Can you work these out from the model? Positions are in its coordinate system, mm. Face numbers are marked on the shaded views. A direction names the side the tool comes from. Give positions to 0.01 mm unless a question says otherwise; leave off trailing zeros. Write each loop counter-clockwise with the first axis right and the second up, starting at its lowest first coordinate (ties: lowest second). Pieces come first, ordered by that corner, then holes.
from build123d import *

# Parameters (mm, degrees)
SKETCH1_R             = 12.7
BOSS_EXTRUDE1_DEPTH   = 6.35
SKETCH2_R             = 6.35
CUT_EXTRUDE1_DEPTH    = 2.38125
SKETCH3_R             = 3.1115
CUT_EXTRUDE2_DEPTH    = 3.175
SKETCH4_R             = 1.190625
CUT_EXTRUDE3_DEPTH    = 4.96875
F_6_32_TAPPED_HOLE1_D = 2.7051
SKETCH7_R             = 1.778
CUT_EXTRUDE4_DEPTH    = 7.35
SKETCH8_R             = 3.175
CUT_EXTRUDE5_DEPTH    = 3.175
CIRPATTERN2_COUNT     = 4
FILLET1_R             = 1.5875


with BuildPart() as part:
    # Sketch1 → Boss-Extrude1 (new body)
    with BuildSketch(Plane(origin=(0, 0, 0), x_dir=(1, 0, 0), z_dir=(0, 1, 0))):
        Circle(SKETCH1_R)
    extrude(amount=BOSS_EXTRUDE1_DEPTH)

    # Sketch2 → Cut-Extrude1 (cut)
    with BuildSketch(Plane(origin=(0, 6.35, 0), x_dir=(1, 0, 0), z_dir=(0, 1, 0))):
        Circle(SKETCH2_R)
    extrude(amount=-CUT_EXTRUDE1_DEPTH, mode=Mode.SUBTRACT)

    # Sketch3 → Cut-Extrude2 (cut)
    with BuildSketch(Plane.XZ):
        Circle(SKETCH3_R)
    extrude(amount=-CUT_EXTRUDE2_DEPTH, mode=Mode.SUBTRACT)

    # Sketch4 → Cut-Extrude3 (cut, through all)
    with BuildSketch(Plane(origin=(0, 3.96875, 0), x_dir=(1, 0, 0), z_dir=(0, 1, 0))):
        Circle(SKETCH4_R)
    extrude(amount=-CUT_EXTRUDE3_DEPTH, mode=Mode.SUBTRACT)

    # #6-32 Tapped Hole1 (through all)
    with Locations(Plane(origin=(0, 6.35, 0), x_dir=(1, 0, 0), z_dir=(0, 1, 0))):
        with Locations((-9.779, 0)):
            f_6_32_tapped_hole1 = Hole(F_6_32_TAPPED_HOLE1_D / 2)

    # Sketch7 → Cut-Extrude4 (cut, through all)
    with BuildSketch(Plane(origin=(0, 6.35, 0), x_dir=(1, 0, 0), z_dir=(0, 1, 0))):
        with Locations((6.914797213, -6.914797213)):
            Circle(SKETCH7_R)
    cut_extrude4 = extrude(amount=-CUT_EXTRUDE4_DEPTH, mode=Mode.SUBTRACT)

    # Sketch8 → Cut-Extrude5 (cut)
    with BuildSketch(Plane.XZ):
        with Locations((6.914797213, 6.914797213)):
            Circle(SKETCH8_R)
    cut_extrude5 = extrude(amount=-CUT_EXTRUDE5_DEPTH, mode=Mode.SUBTRACT)

    # CirPattern2: #6-32 Tapped Hole1, Cut-Extrude4, Cut-Extrude5 ×4 about axis
    cirpattern2_axis = Axis((0, 0, 0), (0, 1, 0))
    for i in range(1, CIRPATTERN2_COUNT):
        add(f_6_32_tapped_hole1.rotate(cirpattern2_axis, i * 360 / CIRPATTERN2_COUNT), mode=Mode.SUBTRACT)
        add(cut_extrude4.rotate(cirpattern2_axis, i * 360 / CIRPATTERN2_COUNT), mode=Mode.SUBTRACT)
        add(cut_extrude5.rotate(cirpattern2_axis, i * 360 / CIRPATTERN2_COUNT), mode=Mode.SUBTRACT)

    # Fillet1
    fillet1_edges = [part.edges().sort_by_distance(p)[0] for p in [
        (7.923120818, 1.5875, 9.925429789),
        (9.925429789, 1.5875, 7.923120818),
        (9.925429789, 1.5875, -7.923120818),
        (7.923120818, 1.5875, -9.925429789),
        (-7.923120818, 1.5875, -9.925429789),
        (-9.925429789, 1.5875, -7.923120818),
        (-9.925429789, 1.5875, 7.923120818),
        (-7.923120818, 1.5875, 9.925429789),
    ]]
    fillet(fillet1_edges, radius=FILLET1_R)


solid = part.part
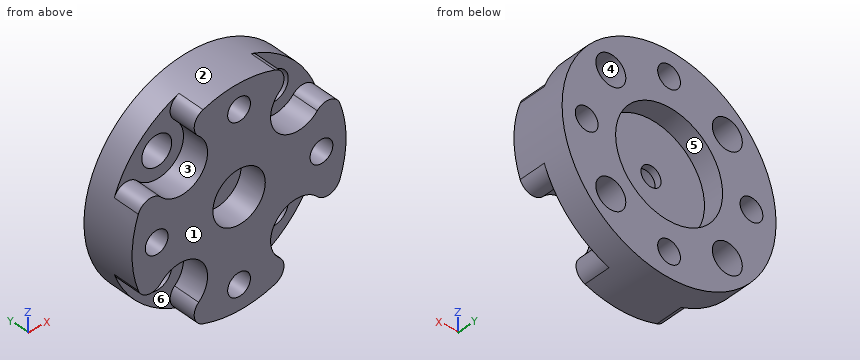
(1) If I drill on L1, parallel to Z at x = 1, y = 3.5; L2, parallel to Z at x = -0.5, y = 2; L3, parallel to Y at x = -9.5, z = 5.25 (3 decimals), over which ranges is the centre line in solid material (lowest first)?
Returned:
L1: z = -12.66 to -10.69, -8.87 to -0.65, 0.65 to 8.87, 10.69 to 12.66
L2: z = -12.69 to -11.04, -8.52 to -3.07, 3.07 to 8.52, 11.04 to 12.69
L3: y = 3.175 to 6.35
(2) Will these pins go through, and if not, where does the flat tip stop? P1, Ø3, axis at x = -6.91, z = -6.91, coming from the +Y side; P2, Ø3, axis at x = 0, z = 0, coming from the -Y side (3 decimals); P3, Ø6.5, axis at x = 9, z = 8, coming from the -Y side; P4, Ø2, axis at y = 3, z = -8.5, coming from the -X side.
Returned:
P1: passes through
P2: stops at y = 3.175
P3: stops at y = 0
P4: stops at x = -10.24
(3) Imagine slicing it at A-A, the plane z = 0. Give the number of separate pieces and of enclosed holes in the cut face, plus the area to 3 significant figures.
Returned:
separate pieces: 4
enclosed holes: 0
area: 75.0 mm2
(4) Imagine slicing it at D-D, the plane z = -5.75. Write out the boundary of the cut face in (x, y) (3 decimals), plus the area to 3 significant figures.
Returned:
outline: (-11.324, 3.175) - (-8.258, 3.175) - (-8.258, 6.35) - (-11.324, 6.35) - close; (-5.571, 3.175) - (-3.961, 3.175) - (-3.961, 0) - (3.961, 0) - (3.961, 3.175) - (5.571, 3.175) - (5.571, 6.35) - (2.694, 6.35) - (2.694, 3.969) - (-2.694, 3.969) - (-2.694, 6.35) - (-5.571, 6.35) - close; (8.258, 3.175) - (11.324, 3.175) - (11.324, 6.35) - (8.258, 6.35) - close
area: 67.2 mm2
(5) For the marked faces 4, 5 and 6, which set-ups out of +Z, -Z, +X, -X, +Y, -Y let a thin tool reach every point of the face, with its end or its side?
Returned:
face 4: +Y, -Y
face 5: +Y
face 6: -Y
(6) If we mould it in two halves opening along Z, with no side actions, what happens to the marked faces 1, 2 and 3? For each: +Z half, -Z half, draft (parallel to the pull), parting line (faces both ways), or undercut.
Returned:
face 1: draft
face 2: parting line
face 3: undercut
